Verification items for the finished model (mm, model axes). Round coordinates to 2 decimals unless told otherwise and drop trailing zeros. Order: outer loops, then holes, each group sorted by start corner. A loop starts at its lowest first (then second) coordinate and runs counter-clockwise, first axis right, second up. Notation, with made-up numbers: (83.25, -24) -> (139.25, -24) arc R35 cw to (139.25, 15) -> close; hole circle Ø8 at (71.25, -18). An arc over 180 degrees is marked (long way). Return JSON: item names as keys, results as strings. Group by question number.
1) Section check C-C on y = -15. Enter the section's corners in (x, z), plus the area to 3 significant figures.
2) Scan lines: L1, parallel to Z at x = 31.5, y = -20; L2, parallel to Y at x = 17, z = 31.5; L3, parallel to Z at x = 24.5, y = -14. Record each from-to range of solid material in increasing order.
3) Section check B-B on x = 31. Enter the section's corners in (y, z), plus the area to 3 significant figures.
4) Section check A-A on y = -20. Enter the section's corners in (x, z), plus the area to 3 significant figures.
5) Depth check by flat-ended pin: pin 1 (16 mm diameter, centred on y = -20, z = 20, fed in from -X); pin 2 (3 mm diameter, centred on x = 21.5, z = 11.5, fed in from -Y); pin 3 (1 mm diameter, centred on x = 19, y = -42, fed in from -Z). Enter the tip coordinate at first touch or a pass-through.
6) Draft check along Y on faces 1 (the flat face through (0, -11, 15)), 2 (the cylindrical face through (19.72, -29.54, 23)), 3 (the flat face through (20, 0, 20)). Enter one of: pulls with the +Y half, pulls with the -Y half, needs draft (parallel to the pull), parting line crosses it, or undercut.
7) Section check D-D on z = 8.5. Enter the section's corners in (x, y).
```python
from build123d import *

# Parameters (mm, degrees)
F0_W     = 40
F0_H     = 40
F1_DEPTH = 40
F2_R     = 10
F3_DEPTH = 40.001


with BuildPart() as f1:
    # F0 (on Front) → F1 (new body)
    with BuildSketch(Plane.XZ):
        with Locations((20, 20)):
            Rectangle(F0_W, F0_H)
    extrude(amount=F1_DEPTH)

    # F2 (on face) → F3 (cut, through all)
    with BuildSketch(Plane(origin=(0, 0, 0), x_dir=(0, -1, 0), z_dir=(-1, 0, 0))):
        with Locations((20, 20)):
            Circle(F2_R)
    extrude(amount=-F3_DEPTH, mode=Mode.SUBTRACT)

    # F4 (on face) → F5 (revolve)
    with BuildSketch(Plane.XZ.offset(40)):
        with BuildLine():
            ThreePointArc((29.395014, 19.543692), (22.16222, 26.88829), (14.929425, 19.543692))
            Line((14.929425, 19.543692), (29.395014, 19.543692))
        make_face()
    revolve(axis=Axis((22.16222, -40, 19.543692), (1, 0, 0)))


solid = f1.part
```
Check result:
{
 "1": {"outline": "(0, 0) -> (40, 0) -> (40, 11.34) -> (0, 11.34) -> close; (0, 28.66) -> (40, 28.66) -> (40, 40) -> (0, 40) -> close", "area": "907 mm^2"},
 "2": {"L1": "0 to 10, 30 to 40", "L2": "-40 to 0", "L3": "0 to 12, 28 to 40"},
 "3": {"outline": "(-40, 0) -> (0, 0) -> (0, 40) -> (-40, 40) -> close; hole circle Ø20 at (-20, 20)", "area": "1,290 mm^2"},
 "4": {"outline": "(0, 0) -> (40, 0) -> (40, 10) -> (0, 10) -> close; (0, 30) -> (40, 30) -> (40, 40) -> (0, 40) -> close", "area": "800 mm^2"},
 "5": {"pin 1": "through", "pin 2": "y = -43.28", "pin 3": "z = 12.96"},
 "6": {"face 1": "needs draft", "face 2": "undercut", "face 3": "pulls with the +Y half"},
 "7": {"outline": "(0, -40) -> (40, -40) -> (40, 0) -> (0, 0) -> close"}
}
